The model under review builds one solid part; all positions refer to its coordinate system, in mm. A direction names the side the tool comes from. Round coordinates to 2 decimals unless told otherwise and drop trailing zeros. Loops run counter-clockwise (first coordinate to the right, second up) from the corner with the lowest first, then second, coordinate; pieces in that order, holes last. Notation, with made-up numbers: M 69.25,-17.75 L 94.25,-17.75 A23 cw 94.25,21.25 Z; hole C 56.5,-7.75 d9. An arc over 180 degrees is marked long. Answer as a JSON object with one key per item and string values. Group by question number.
Item 1: Consider section C-C (x = 2.5). Give the boundary of the cut face in (y, z), and give its area (3 significant figures).
Item 2: To check wall thickness, follow line 1 (X direction, y = 6.5, z = 20); line 2 (X direction, y = 6.15, z = -6); line 3 (X direction, y = 4.5, z = 24.5). State the ranges of each line that lie inside material, in increasing order.
Item 3: Tool access review of faces 3 (the face through (9.3, 4, -18.5)), 4 (the face through (7.05, 5, 18)), 5 (the face through (-3.55, 5, 0)): name each direction out of +Z, -Z, +X, -X, +Y, -Y from which nothing blocks a thin tool from reaching the whole face with its end or side.
Item 4: Insertion check: P1, Ø2.5, axis at x = -9.25, z = 20, coming from the -Y side; P2, Ø2, axis at y = 4.5, z = -0.5, coming from the +X side; P3, Ø1.5, axis at y = 5, z = -24.5, coming from the +X side. Each pin has a flat end and moves straight along its axis. Give the tip position at first contact, or say it passes through.
Item 5: Consider section A-A (x = -6). Give the boundary of the cut face in (y, z), and give its area (3 significant figures).
Item 6: Consider section D-D (z = -25). Give the boundary of the cut face in (x, y), and give its area (3 significant figures).
Item 7: Consider section B-B (z = -12.5). Give the boundary of the cut face in (x, y), and give its area (3 significant figures).
Item 8: The part is to be moulded in two halves that separate along Z. For faces 1 (the face through (0, 5, -31.5)), 2 (the face through (7.51, 4.42, 5.14)), say which applies: +Z half, -Z half, draft (parallel to the pull), parting line (faces both ways), or undercut.
```python
from build123d import *

# Parameters (mm, degrees)
SKETCH_4_W           = 23.5
SKETCH_4_H           = 63
EXTRUDE_1_DEPTH      = 7
SKETCH_5_R           = 1.75
CUT_EXTRUDE_1_DEPTH  = 40.918667312
SKETCH_5_3_R         = 3
CUT_EXTRUDE_4_DEPTH  = 2.7
CUT_EXTRUDE_START    = -20.8
SKETCH_5_4_R         = 3
CUT_EXTRUDE_5_DEPTH  = 2.7
SKETCH_5_5_R         = 3
CUT_EXTRUDE_6_DEPTH  = 2.7
SKETCH_5_6_R         = 3
CUT_EXTRUDE_7_DEPTH  = 2.7
SKETCH_6_R           = 1.5
SKETCH_6_R_2         = 1
CUT_EXTRUDE_2_DEPTH  = 5
SKETCH_6_2_R         = 1
CUT_EXTRUDE_3_DEPTH  = 35.341119667
CUT_EXTRUDE_8_DEPTH  = 6
CUT_EXTRUDE_START_2  = -1
SKETCH_12_R          = 5.75
CUT_EXTRUDE_9_DEPTH  = 3.4
CUT_EXTRUDE_START_3  = 0.4
SKETCH_13_R          = 8.25
CUT_EXTRUDE_10_DEPTH = 2
SKETCH_14_R          = 3.25
CUT_EXTRUDE_11_DEPTH = 4
CUT_EXTRUDE_START_4  = -4.7
SKETCH_15_R          = 1
CUT_EXTRUDE_12_DEPTH = 3
CUT_EXTRUDE_START_5  = -13.7
SKETCH_15_2_R        = 1
CUT_EXTRUDE_15_DEPTH = 3
SKETCH_16_R          = 5.75
CUT_EXTRUDE_13_DEPTH = 3.4
SKETCH_17_W          = 23.5
SKETCH_17_H          = 63
CUT_EXTRUDE_14_DEPTH = 3


with BuildPart() as part:
    # 草图4 → 凸台-拉伸1 (new body)
    with BuildSketch(Plane(origin=(0, 0, 0), x_dir=(1, 0, 0), z_dir=(0, 1, 0))):
        Rectangle(SKETCH_4_W, SKETCH_4_H)
    extrude(amount=EXTRUDE_1_DEPTH)

    # 草图5 → 切除-拉伸1 (cut, through all)
    with BuildSketch(Plane(origin=(11.75, 0, 0), x_dir=(0, 0, -1), z_dir=(1, 0, 0))):
        with Locations((-25, 7)):
            Circle(SKETCH_5_R)
        with Locations((0, 7)):
            Circle(SKETCH_5_R)
        with Locations((25, 7)):
            Circle(SKETCH_5_R)
    extrude(amount=-CUT_EXTRUDE_1_DEPTH, mode=Mode.SUBTRACT)

    # 草图5<3> → 切除-拉伸4 (cut)
    with BuildSketch(Plane(origin=(11.75, 0, 0), x_dir=(0, 0, -1), z_dir=(1, 0, 0))):
        with Locations((-25, 7)):
            Circle(SKETCH_5_3_R)
        with Locations((25, 7)):
            Circle(SKETCH_5_3_R)
    extrude(amount=-CUT_EXTRUDE_4_DEPTH, mode=Mode.SUBTRACT)

    # 草图5<4> → 切除-拉伸5 (cut)
    with BuildSketch(Plane(origin=(11.75, 0, 0), x_dir=(0, 0, -1), z_dir=(1, 0, 0)).offset(CUT_EXTRUDE_START)):
        with Locations((-25, 7)):
            Circle(SKETCH_5_4_R)
        with Locations((25, 7)):
            Circle(SKETCH_5_4_R)
    extrude(amount=-CUT_EXTRUDE_5_DEPTH, mode=Mode.SUBTRACT)

    # 草图5<5> → 切除-拉伸6 (cut)
    with BuildSketch(Plane(origin=(11.75, 0, 0), x_dir=(0, 0, -1), z_dir=(1, 0, 0))):
        with Locations((0, 7)):
            Circle(SKETCH_5_5_R)
    extrude(amount=-CUT_EXTRUDE_6_DEPTH, mode=Mode.SUBTRACT)

    # 草图5<6> → 切除-拉伸7 (cut)
    with BuildSketch(Plane(origin=(11.75, 0, 0), x_dir=(0, 0, -1), z_dir=(1, 0, 0)).offset(CUT_EXTRUDE_START)):
        with Locations((0, 7)):
            Circle(SKETCH_5_6_R)
    extrude(amount=-CUT_EXTRUDE_7_DEPTH, mode=Mode.SUBTRACT)

    # 草图6 → 切除-拉伸2 (cut)
    # profile 1 of 8: a face of its own
    with BuildSketch(Plane.XZ):
        with Locations(Location((-9.25, 6, 0), (0, 0, 270))):
            Circle(SKETCH_6_R)
        with Locations(Location((-9.25, 6, 0), (0, 0, 270))):
            Circle(SKETCH_6_R_2, mode=Mode.SUBTRACT)
    # profile 2 of 8: a face of its own
    with BuildSketch(Plane.XZ):
        with Locations(Location((9.25, 6, 0), (0, 0, 270))):
            Circle(SKETCH_6_R)
        with Locations(Location((9.25, 6, 0), (0, 0, 270))):
            Circle(SKETCH_6_R_2, mode=Mode.SUBTRACT)
    # profile 3 of 8: a face of its own
    with BuildSketch(Plane.XZ):
        with Locations(Location((-9.25, -20, 0), (0, 0, 270))):
            Circle(SKETCH_6_R)
        with Locations(Location((-9.25, -20, 0), (0, 0, 270))):
            Circle(SKETCH_6_R_2, mode=Mode.SUBTRACT)
    # profile 4 of 8: a face of its own
    with BuildSketch(Plane.XZ):
        with Locations(Location((9.25, -20, 0), (0, 0, 270))):
            Circle(SKETCH_6_R)
        with Locations(Location((9.25, -20, 0), (0, 0, 270))):
            Circle(SKETCH_6_R_2, mode=Mode.SUBTRACT)
    # profile 5 of 8: a face of its own
    with BuildSketch(Plane.XZ):
        with Locations(Location((-9.25, 20, 0), (0, 0, 270))):
            Circle(SKETCH_6_R)
        with Locations(Location((-9.25, 20, 0), (0, 0, 270))):
            Circle(SKETCH_6_R_2, mode=Mode.SUBTRACT)
    # profile 6 of 8: a face of its own
    with BuildSketch(Plane.XZ):
        with Locations(Location((9.25, 20, 0), (0, 0, 270))):
            Circle(SKETCH_6_R)
        with Locations(Location((9.25, 20, 0), (0, 0, 270))):
            Circle(SKETCH_6_R_2, mode=Mode.SUBTRACT)
    # profile 7 of 8: a face of its own
    with BuildSketch(Plane.XZ):
        with Locations(Location((-9.25, -6, 0), (0, 0, 270))):
            Circle(SKETCH_6_R)
        with Locations(Location((-9.25, -6, 0), (0, 0, 270))):
            Circle(SKETCH_6_R_2, mode=Mode.SUBTRACT)
    # profile 8 of 8: a face of its own
    with BuildSketch(Plane.XZ):
        with Locations(Location((9.25, -6, 0), (0, 0, 270))):
            Circle(SKETCH_6_R)
        with Locations(Location((9.25, -6, 0), (0, 0, 270))):
            Circle(SKETCH_6_R_2, mode=Mode.SUBTRACT)
    extrude(amount=-CUT_EXTRUDE_2_DEPTH, mode=Mode.SUBTRACT)

    # 草图6<2> → 切除-拉伸3 (cut, through all)
    with BuildSketch(Plane.XZ):
        with Locations(Location((-9.25, -20, 0), (0, 0, 270))):
            Circle(SKETCH_6_2_R)
        with Locations(Location((9.25, -20, 0), (0, 0, 270))):
            Circle(SKETCH_6_2_R)
        with Locations(Location((-9.25, 20, 0), (0, 0, 270))):
            Circle(SKETCH_6_2_R)
        with Locations(Location((9.25, 20, 0), (0, 0, 270))):
            Circle(SKETCH_6_2_R)
        with Locations(Location((9.25, -6, 0), (0, 0, 270))):
            Circle(SKETCH_6_2_R)
        with Locations(Location((-9.25, -6, 0), (0, 0, 270))):
            Circle(SKETCH_6_2_R)
        with Locations(Location((-9.25, 6, 0), (0, 0, 270))):
            Circle(SKETCH_6_2_R)
        with Locations(Location((9.25, 6, 0), (0, 0, 270))):
            Circle(SKETCH_6_2_R)
    extrude(amount=-CUT_EXTRUDE_3_DEPTH, mode=Mode.SUBTRACT)

    # 草图10 → 切除-拉伸8 (cut)
    with BuildSketch(Plane(origin=(0, 7, 0), x_dir=(1, 0, 0), z_dir=(0, 1, 0))):
        Polygon((-8.75, 2.6), (-8.75, -2.6), (-6.75, -2.6), (-6.75, -5.75), (-3.55, -5.75), (-3.55, 5.75), (-6.75, 5.75), (-6.75, 2.6), align=None)
    extrude(amount=-CUT_EXTRUDE_8_DEPTH, mode=Mode.SUBTRACT)

    # 草图12 → 切除-拉伸9 (cut)
    with BuildSketch(Plane(origin=(9.05, 0, 0), x_dir=(0, 0, -1), z_dir=(1, 0, 0)).offset(CUT_EXTRUDE_START_2)):
        with Locations((0, 7)):
            Circle(SKETCH_12_R)
    extrude(amount=-CUT_EXTRUDE_9_DEPTH, mode=Mode.SUBTRACT)

    # 草图13 → 切除-拉伸10 (cut)
    with BuildSketch(Plane(origin=(4.65, 0, 0), x_dir=(0, 0, -1), z_dir=(1, 0, 0)).offset(CUT_EXTRUDE_START_3)):
        with Locations((-12.5, 7)):
            Circle(SKETCH_13_R)
        with Locations((12.5, 7)):
            Circle(SKETCH_13_R)
    extrude(amount=CUT_EXTRUDE_10_DEPTH, mode=Mode.SUBTRACT)

    # 草图14 → 切除-拉伸11 (cut)
    with BuildSketch(Plane(origin=(5.05, 0, 0), x_dir=(0, 0, -1), z_dir=(1, 0, 0))):
        with Locations((-12.5, 7)):
            Circle(SKETCH_14_R)
        with Locations((12.5, 7)):
            Circle(SKETCH_14_R)
    extrude(amount=-CUT_EXTRUDE_11_DEPTH, mode=Mode.SUBTRACT)

    # 草图15 → 切除-拉伸12 (cut)
    with BuildSketch(Plane(origin=(11.75, 0, 0), x_dir=(0, 0, -1), z_dir=(1, 0, 0)).offset(CUT_EXTRUDE_START_4)):
        with Locations((-12.5, 7)):
            Circle(SKETCH_15_R)
        with Locations((12.5, 7)):
            Circle(SKETCH_15_R)
    extrude(amount=CUT_EXTRUDE_12_DEPTH, mode=Mode.SUBTRACT)

    # 草图15<2> → 切除-拉伸15 (cut)
    with BuildSketch(Plane(origin=(11.75, 0, 0), x_dir=(0, 0, -1), z_dir=(1, 0, 0)).offset(CUT_EXTRUDE_START_5)):
        with Locations((-12.5, 7)):
            Circle(SKETCH_15_2_R)
        with Locations((12.5, 7)):
            Circle(SKETCH_15_2_R)
    extrude(amount=CUT_EXTRUDE_15_DEPTH, mode=Mode.SUBTRACT)

    # 草图16 → 切除-拉伸13 (cut)
    with BuildSketch(Plane.ZY.offset(-7.05)):
        with Locations((25, 7)):
            Circle(SKETCH_16_R)
        with Locations((-25, 7)):
            Circle(SKETCH_16_R)
    extrude(amount=CUT_EXTRUDE_13_DEPTH, mode=Mode.SUBTRACT)

    # 草图17 → 切除-拉伸14 (cut)
    with BuildSketch(Plane.XZ):
        Rectangle(SKETCH_17_W, SKETCH_17_H)
    extrude(amount=-CUT_EXTRUDE_14_DEPTH, mode=Mode.SUBTRACT)


solid = part.part
```
Geometry results:
{
 "1": {"outline": "M 3,-31.5 L 7,-31.5 L 7,-26.75 A1.75 cw 7,-23.25 L 7,-15.75 A3.25 cw 7,-9.25 L 7,-1.75 A1.75 cw 7,1.75 L 7,9.25 A3.25 cw 7,15.75 L 7,23.25 A1.75 cw 7,26.75 L 7,31.5 L 3,31.5 Z", "area": "204 mm^2"},
 "2": {"line 1": "x = -11.75 to -10.25, -8.25 to 3.65, 7.05 to 8.25, 10.25 to 11.75", "line 2": "x = -11.75 to -10.25, -8.25 to 5.05, 7.05 to 8.25, 10.25 to 11.75", "line 3": "x = -9.05 to 3.65, 7.05 to 9.05"},
 "3": {"face 3": "-Y", "face 4": "+Y", "face 5": "+Y, -Y"},
 "4": {"P1": "stops at y = 5", "P2": "stops at x = 11.75", "P3": "stops at x = 9.05"},
 "5": {"outline": "M 3,-31.5 L 7,-31.5 L 7,-26.75 A1.75 cw 7,-23.25 L 7,-5.75 L 3,-5.75 Z; M 3,5.75 L 7,5.75 L 7,23.25 A1.75 cw 7,26.75 L 7,31.5 L 3,31.5 Z", "area": "196 mm^2"},
 "6": {"outline": "M -11.75,3 L 3.65,3 L 3.65,5.25 L -9.05,5.25 L -9.05,4 L -11.75,4 Z; M 7.05,3 L 11.75,3 L 11.75,4 L 9.05,4 L 9.05,5.25 L 7.05,5.25 Z", "area": "38.5 mm^2"},
 "7": {"outline": "M -11.75,3 L 5.05,3 L 5.05,3.75 L 1.05,3.75 L 1.05,6 L -1.95,6 L -1.95,7 L -11.75,7 Z; M 7.05,3 L 11.75,3 L 11.75,7 L 10.05,7 L 10.05,6 L 7.05,6 Z", "area": "67.0 mm^2"},
 "8": {"face 1": "-Z half", "face 2": "undercut"}
}
